Can you work these out from the drawing? Everything is in mm from the part's minimum corner. Give positions to 0.01 mm unless a question says otherwise; leave off trailing zeros. Write each loop counter-clockwise with the first axis right and the second up, starting at its lowest first coordinate (ties: lowest second). Pieces come first, ordered by that corner, then holes. Notation, with made-up numbers: (80, 7.25) - (135, 7.25) arc R20 ccw to (135, 14.25) - close; hole circle Ø1 at (74.5, 21). An arc over 180 degrees is marked (long way). Write each question's results on one line, items separated by ' | '. Start each with the question number.
Item 1: Suppose I cut it at B-B on z = 128. List the corners of the cut face in (x, y) for me.
Item 2: Will these pins go through, and if not, where does the flat tip stop? P1, Ø15, axis at y = 1276.5, z = 393, coming from the -X side; P2, Ø25, axis at x = 20, y = 899.5, coming from the -Z side.
Item 3: Suppose I cut it at C-C on x = 230. List the corners of the cut face in (y, z) for me.
Item 4: Suppose I cut it at A-A on y = 289. List the corners of the cut face in (x, z) for me.
Item 5: Please list where this line runs through material, in increasing order: line 1 along Z through (x, y) = (27.5, 683).
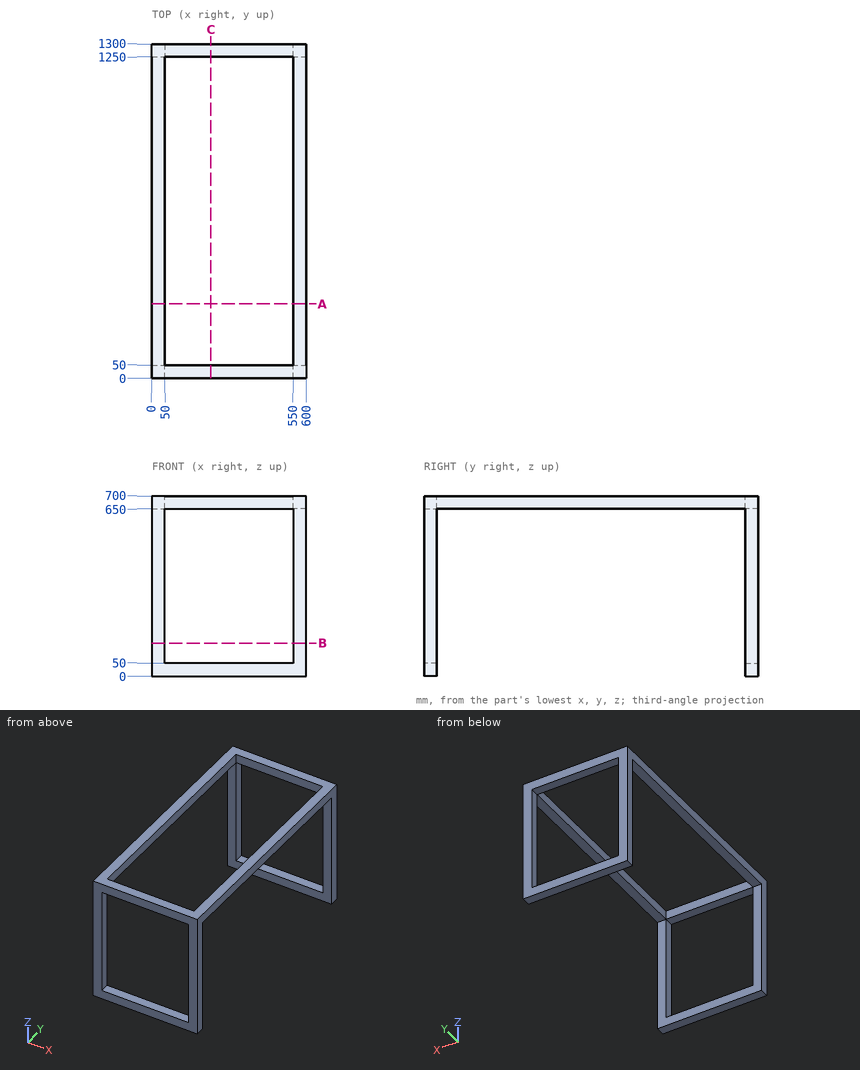
Checked values:
1) outline: (0, 0) - (50, 0) - (50, 50) - (0, 50) - close; (0, 1250) - (50, 1250) - (50, 1300) - (0, 1300) - close; (550, 0) - (600, 0) - (600, 50) - (550, 50) - close; (550, 1250) - (600, 1250) - (600, 1300) - (550, 1300) - close
2) P1: stops at x = 0 | P2: stops at z = 650
3) outline: (0, 0) - (50, 0) - (50, 50) - (0, 50) - close; (0, 650) - (50, 650) - (50, 700) - (0, 700) - close; (1250, 0) - (1300, 0) - (1300, 50) - (1250, 50) - close; (1250, 650) - (1300, 650) - (1300, 700) - (1250, 700) - close
4) outline: (0, 650) - (50, 650) - (50, 700) - (0, 700) - close; (550, 650) - (600, 650) - (600, 700) - (550, 700) - close
5) line 1: z = 650 to 700
